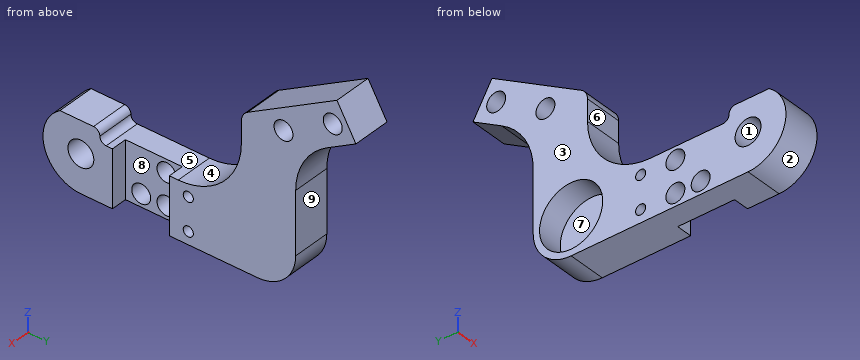
from build123d import *

# Parameters (mm, degrees)
SKETCH1_R                   = 2.05
SKETCH1_R_2                 = 1.5
BOSS_EXTRUDE1_DEPTH         = 6
FILLET1_START               = -1
FILLET1_DEPTH               = 8
FILLET1_2_DEPTH             = 6
TAP_DRILL_FOR_M2X0_4_TAP1_D = 1.6
SKETCH4_W                   = 9
SKETCH4_H                   = 9
CUT_EXTRUDE1_DEPTH          = 2.5
SKETCH5_R                   = 5
CUT_EXTRUDE2_DEPTH          = 4


with BuildPart() as part:
    # Sketch1 → Boss-Extrude1 (new body)
    with BuildSketch(Plane(origin=(0, 0, 0), x_dir=(0, 0, -1), z_dir=(1, 0, 0))):
        with BuildLine():
            Line((6, 0), (6, 28))
            ThreePointArc((6, 28), (4.242640687, 32.242640687), (0, 34))
            Line((0, 34), (-9.814222224, 34))
            ThreePointArc((-9.814222224, 34), (-14.814222224, 35.339745962), (-18.474476262, 39))
            Line((-18.474476262, 39), (-21.089872981, 43.53))
            Line((-21.089872981, 43.53), (-26.286025404, 40.53))
            Line((-26.286025404, 40.53), (-18.131025404, 26.405125664))
            ThreePointArc((-18.131025404, 26.405125664), (-17.398974596, 25.673074857), (-16.398974596, 25.405125664))
            Line((-16.398974596, 25.405125664), (-13, 25.405125664))
            ThreePointArc((-13, 25.405125664), (-5.928932188, 22.476193476), (-3, 15.405125664))
            Line((-3, 15.405125664), (-3, 3))
            Line((-3, 3), (-5, 3))
            Line((-5, 3), (-5, -3.31662479))
            ThreePointArc((-5, -3.31662479), (1.732050808, -5.744562647), (6, 0))
        make_face()
        Circle(SKETCH1_R, mode=Mode.SUBTRACT)
        with Locations((-22.437949192, 39.864936491)):
            Circle(SKETCH1_R_2, mode=Mode.SUBTRACT)
        with Locations((-17.937949192, 32.070707856)):
            Circle(SKETCH1_R_2, mode=Mode.SUBTRACT)
        with Locations((-1, 11.5)):
            Circle(SKETCH1_R_2, mode=Mode.SUBTRACT)
        with Locations((4, 11.5)):
            Circle(SKETCH1_R_2, mode=Mode.SUBTRACT)
        with Locations((4, 7.5)):
            Circle(SKETCH1_R_2, mode=Mode.SUBTRACT)
    extrude(amount=BOSS_EXTRUDE1_DEPTH)

    # Fillet1: read off the stored shape, not the designer's step
    # Fillet1 outline → Fillet1 (cut)
    with BuildSketch(Plane.YZ.offset(FILLET1_START)):
        with BuildLine():
            ThreePointArc((2, 5), (2.707106781, 4.707106781), (3, 4))
            Line((3, 4), (3, 5))
            Line((3, 5), (2, 5))
        make_face()
    extrude(amount=FILLET1_DEPTH, mode=Mode.SUBTRACT)

    # Fillet1 2 outline → Fillet1 2 (add)
    with BuildSketch(Plane.YZ):
        with BuildLine():
            ThreePointArc((4, 3), (3.292893219, 3.292893219), (3, 4))
            Line((3, 4), (3, 3))
            Line((3, 3), (4, 3))
        make_face()
    extrude(amount=FILLET1_2_DEPTH)

    # Tap Drill for M2x0.4 Tap1 (through all)
    with Locations(Plane(origin=(6, 0, 0), x_dir=(0, 0, -1), z_dir=(1, 0, 0))):
        with Locations((-1.2, 17), (4, 17)):
            Hole(TAP_DRILL_FOR_M2X0_4_TAP1_D / 2)

    # Sketch4 → Cut-Extrude1 (cut)
    with BuildSketch(Plane.ZY.offset(-6)):
        with Locations((-1.5, 9.5)):
            Rectangle(SKETCH4_W, SKETCH4_H)
    extrude(amount=CUT_EXTRUDE1_DEPTH, mode=Mode.SUBTRACT)

    # Sketch5 → Cut-Extrude2 (cut)
    with BuildSketch(Plane(origin=(0, 0, 0), x_dir=(0, 0, -1), z_dir=(1, 0, 0))):
        with Locations((0, 28)):
            Circle(SKETCH5_R)
    extrude(amount=CUT_EXTRUDE2_DEPTH, mode=Mode.SUBTRACT)


solid = part.part
Could you check a few things on this model? Use its own coordinates, in mm. Face numbers are marked on the shaded views. A direction names the side the tool comes from. Give positions to 0.01 mm unless a question says otherwise; leave off trailing zeros. Order: outer loops, then holes, each group sorted by start corner. A loop starts at its lowest first (then second) coordinate and runs counter-clockwise, first axis right, second up.
Item 1: If we section it at D-D, the plane x = 2.2: Count the separate pieces of the cut face and the enclosed holes in it, plus the area to 3 significant figures.
Item 2: I need wall thicknesses on line 1 (Z direction, x = 2.55, y = 11); line 2 (Y direction, x = 1.65, z = 1.5); line 3 (Y direction, x = 2.95, z = 17). Which ranges of each line are inside material? Lowest first, please.
Item 3: I'm going to push flat-ended pins straight in: pin 1 (3 mm diameter, centred on x = 2.5, y = 7, fed in from +Z); pin 2 (4 mm diameter, centred on y = 11.5, z = 1, fed in from +X); pin 3 (2.5 mm diameter, centred on y = 32.07, z = 17.94, fed in from -X); pin 4 (8 mm diameter, centred on y = 28, z = 0, fed in from -X). Where does each tip first touch, or does it pass through?
Item 4: For the marked faces 5, 6, 7, 8 and 9, which set-ups out of +Z, -Z, +X, -X, +Y, -Y let a thin tool reach every point of the face, with its end or its side?
Item 5: If we section it at B-B, the plane y = 31.5: Write out the boundary of the cut face in (x, z).
Item 6: If we section it at A-A, the plane y = 11.5: Write out the boundary of the cut face in (x, z).
Item 7: If we mould it in two halves opening along Y, with no side actions, what happens to the marked faces 1, 2, 3 and 4? For each: pulls with the +Y half, pulls with the -Y half, needs draft (parallel to the pull), parting line crosses it, or undercut.
Item 8: If we section it at C-C, the plane z = 1.2: Write out the boundary of the cut face in (x, y).
Values:
1. separate pieces: 1
1. enclosed holes: 9
1. area: 456 mm2
2. line 1: z = -6 to -5.41, -2.59 to -0.41, 2.41 to 3
2. line 2: y = -5.81 to -1.4, 1.4 to 10.09, 12.91 to 16.26, 17.74 to 23.23, 32.77 to 34
2. line 3: y = 25.5 to 30.9, 33.24 to 37.05
3. pin 1: stops at z = 3
3. pin 2: stops at x = 3.5
3. pin 3: passes through
3. pin 4: stops at x = 4
4. face 5: +Z, +X, -X
4. face 6: +Z, +X, -X, -Y
4. face 7: -X
4. face 8: +Z, -Z, +X
4. face 9: -Z, +X, -X, +Y
5. outline: (0, -4.87) - (6, -4.87) - (6, 16.55) - (0, 16.55) - (0, 3.57) - (4, 3.57) - (4, -3.57) - (0, -3.57) - close; (0, 19.33) - (6, 19.33) - (6, 21.07) - (0, 21.07) - close
6. outline: (0, -6) - (3.5, -6) - (3.5, -5.5) - (0, -5.5) - close; (0, -2.5) - (3.5, -2.5) - (3.5, -0.5) - (0, -0.5) - close; (0, 2.5) - (3.5, 2.5) - (3.5, 3) - (0, 3) - close
7. face 1: undercut
7. face 2: pulls with the -Y half
7. face 3: needs draft
7. face 4: undercut
8. outline: (0, -5.88) - (6, -5.88) - (6, -1.66) - (0, -1.66) - close; (0, 1.66) - (6, 1.66) - (6, 5) - (3.5, 5) - (3.5, 10.01) - (0, 10.01) - close; (0, 12.99) - (3.5, 12.99) - (3.5, 14) - (6, 14) - (6, 16.2) - (0, 16.2) - close; (0, 17.8) - (6, 17.8) - (6, 34) - (0, 34) - (0, 32.85) - (4, 32.85) - (4, 23.15) - (0, 23.15) - close
